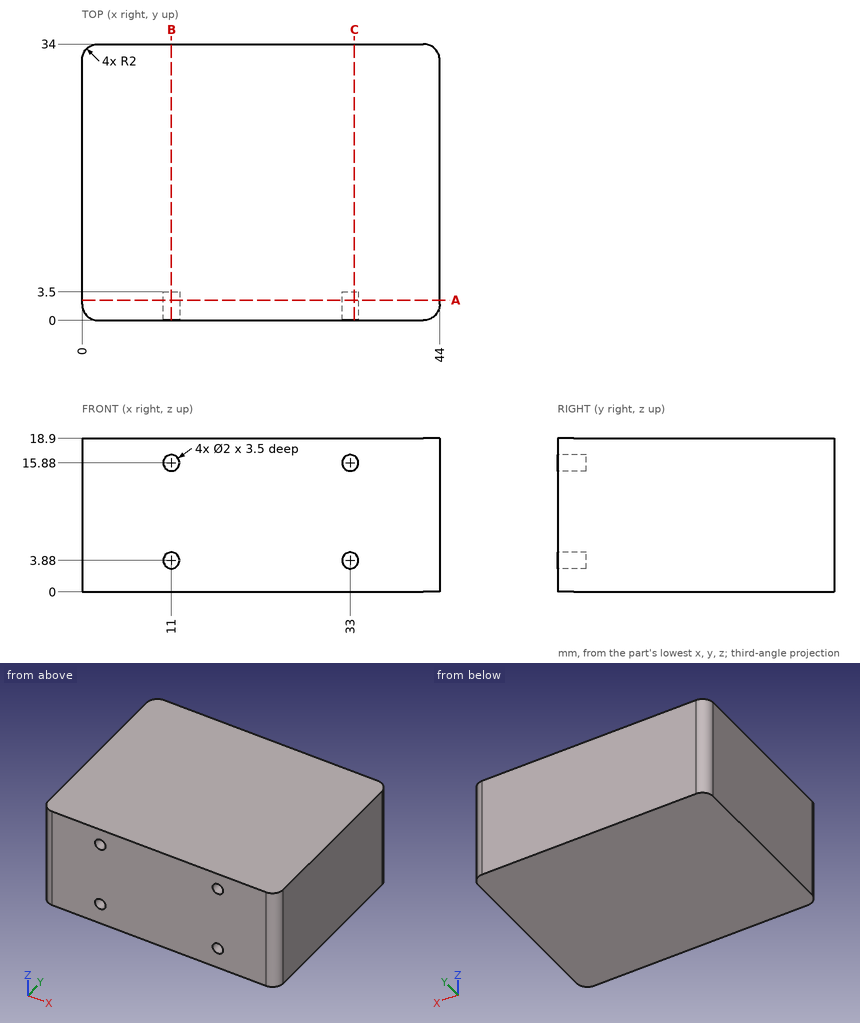
Print and shaded views of the part. All mm, measured from the part's lowest x, y and z. Give positions to 0.01 mm unless a question says otherwise; leave off trailing zeros. Loops run counter-clockwise (first coordinate to the right, second up) from the corner with the lowest first, then second, coordinate; pieces in that order, holes last. Notation, with made-up numbers: M -16.5,54 L -5.5,54 A4 cw -5.5,60 Z; hole C 15.5,-25 d9. An arc over 180 degrees is marked long. Write each question's results on one line, items separated by ' | '.
Q1. Band-saw the part on A-A on y = 2.5. Write the cut outline in (x, z), and give its area (3 significant figures).
Geometry check:
outline: M 0,0 L 44,0 L 44,18.9 L 0,18.9 Z; hole C 11,3.88 d2; hole C 11,15.88 d2; hole C 33,3.88 d2; hole C 33,15.88 d2 | area: 819 mm²
Q2. Probe probe 1 along X at (y, z) = (2.55, 15.88); probe 2 along Z at (x, y) = (33, 1); probe 3 along X at (y, z) = (3, 4.25). List the from-to ranges inside material, lowest first.
Geometry check:
probe 1: x = 0 to 10, 12 to 32, 34 to 44 | probe 2: z = 0 to 2.88, 4.88 to 14.88, 16.88 to 18.9 | probe 3: x = 0 to 10.07, 11.93 to 32.07, 33.93 to 44
Q3. Band-saw the part on B-B on x = 11. Write the cut outline in (y, z), and give its area (3 significant figures).
Geometry check:
outline: M 0,0 L 34,0 L 34,18.9 L 0,18.9 L 0,16.88 L 3.5,16.88 L 3.5,14.88 L 0,14.88 L 0,4.88 L 3.5,4.88 L 3.5,2.88 L 0,2.88 Z | area: 629 mm²
Q4. Band-saw the part on C-C on x = 33.5. Write the cut outline in (y, z).
Geometry check:
outline: M 0,0 L 34,0 L 34,18.9 L 0,18.9 L 0,16.75 L 3.5,16.75 L 3.5,15.01 L 0,15.01 L 0,4.75 L 3.5,4.75 L 3.5,3.01 L 0,3.01 Z
Q5. Flat gauge pins, fed straight in: P1, Ø1.2, axis at x = 33, z = 15.88, coming from the -Y side; P2, Ø8, axis at y = 19, z = 2.5, coming from the -X side. Where does each tip first touch, or does it go through?
Geometry check:
P1: stops at y = 3.5 | P2: stops at x = 0
